```python
from build123d import *

# Parameters (mm, degrees)
F0_R      = 1.778
F1_DEPTH  = 4
F2_R      = 38
F2_R_2    = 34.25
F3_DEPTH  = 15.24
F4_R      = 33.9471
F4_R_2    = 31
F5_DEPTH  = 1.27
F7_DEPTH  = 5.08
F8_R      = 3.81221
F8_R_2    = 3.881316
F8_R_3    = 3.942619
F8_R_4    = 3.925346
F9_DEPTH  = 1.5
F10_R     = 1.778
F11_DEPTH = 25.4


with BuildPart() as f1:
    # F0 (on Top) → F1 (new body)
    with BuildSketch(Plane.XY):
        Polygon((38.268343, -38.268343), (54.11961, 0), (38.268343, 38.268343), (0, 54.11961), (-38.268343, 38.268343), (-54.11961, 0), (-38.268343, -38.268343), (0, -54.11961), align=None)
        with Locations((0, -45.129232)):
            Circle(F0_R, mode=Mode.SUBTRACT)
        with Locations((-45.129232, 0)):
            Circle(F0_R, mode=Mode.SUBTRACT)
        with Locations((45.129232, 0)):
            Circle(F0_R, mode=Mode.SUBTRACT)
        with Locations((0, 45.129232)):
            Circle(F0_R, mode=Mode.SUBTRACT)
    extrude(amount=F1_DEPTH)

    # F2 (on Top) → F3 (join)
    with BuildSketch(Plane.XY):
        Circle(F2_R)
        Circle(F2_R_2, mode=Mode.SUBTRACT)
    extrude(amount=F3_DEPTH)

    # F4 (on face) → F5 (join)
    with BuildSketch(Plane.XY.offset(4)):
        Circle(F4_R)
        Circle(F4_R_2, mode=Mode.SUBTRACT)
    extrude(amount=F5_DEPTH)

    # F6 (on face) → F7 (join)
    with BuildSketch(Plane.XY.offset(4)):
        Polygon((7.838351, 13.74736), (-7.838351, 13.74736), (-7.838351, 11.297162), (-7.838351, 7.838351), (-11.297162, 7.838351), (-13.74736, 7.838351), (-13.74736, -7.838351), (-11.117557, -7.838351), (-7.838351, -7.838351), (-7.838351, -11.117557), (-7.838351, -13.74736), (7.838351, -13.74736), (7.838351, -11.297162), (7.838351, -7.838351), (11.297162, -7.838351), (13.74736, -7.838351), (13.74736, 7.838351), (11.117557, 7.838351), (7.838351, 7.838351), (7.838351, 11.117557), align=None)
        with BuildLine():
            ThreePointArc((-5.298351, 6.12736), (-3.810454, 9.719462), (-0.218351, 11.20736))
            Line((-0.218351, 11.20736), (0.218351, 11.20736))
            ThreePointArc((0.218351, 11.20736), (3.810454, 9.719462), (5.298351, 6.12736))
            Line((5.298351, 6.12736), (5.298351, 5.298351))
            Line((5.298351, 5.298351), (6.12736, 5.298351))
            ThreePointArc((6.12736, 5.298351), (9.719462, 3.810454), (11.20736, 0.218351))
            Line((11.20736, 0.218351), (11.20736, -0.218351))
            ThreePointArc((11.20736, -0.218351), (9.719462, -3.810454), (6.12736, -5.298351))
            Line((6.12736, -5.298351), (5.298351, -5.298351))
            Line((5.298351, -5.298351), (5.298351, -6.12736))
            ThreePointArc((5.298351, -6.12736), (3.810454, -9.719462), (0.218351, -11.20736))
            Line((0.218351, -11.20736), (-0.218351, -11.20736))
            ThreePointArc((-0.218351, -11.20736), (-3.810454, -9.719462), (-5.298351, -6.12736))
            Line((-5.298351, -6.12736), (-5.298351, -5.298351))
            Line((-5.298351, -5.298351), (-6.12736, -5.298351))
            ThreePointArc((-6.12736, -5.298351), (-9.719462, -3.810454), (-11.20736, -0.218351))
            Line((-11.20736, -0.218351), (-11.20736, 0.218351))
            ThreePointArc((-11.20736, 0.218351), (-9.719462, 3.810454), (-6.12736, 5.298351))
            Line((-6.12736, 5.298351), (-5.298351, 5.298351))
            Line((-5.298351, 5.298351), (-5.298351, 6.12736))
        make_face(mode=Mode.SUBTRACT)
    extrude(amount=F7_DEPTH)

    # F8 (on face) → F9 (join)
    with BuildSketch(Plane.XY.offset(4)):
        with Locations((0, 45.151103)):
            Circle(F8_R)
        with Locations((-45.181099, 0)):
            Circle(F8_R_2)
        with Locations((0, -45.120213)):
            Circle(F8_R_3)
        with Locations((45.201581, 0)):
            Circle(F8_R_4)
    extrude(amount=F9_DEPTH)

    # F10 (on face) → F11 (cut)
    with BuildSketch(Plane(origin=(0, 0, 0), x_dir=(1, 0, 0), z_dir=(0, 0, -1))):
        with Locations((45.129232, 0)):
            Circle(F10_R)
        with Locations((0, -45.129232)):
            Circle(F10_R)
        with Locations((-45.129232, 0)):
            Circle(F10_R)
        with Locations((0, 45.129232)):
            Circle(F10_R)
    extrude(amount=-F11_DEPTH, mode=Mode.SUBTRACT)


solid = f1.part
```
The model under review builds one solid part; all positions refer to its coordinate system, in mm. A direction names the side the tool comes from. Coordinates: 2 decimals unless noted, no trailing zeros. Write each loop counter-clockwise with the first axis right and the second up, starting at its lowest first coordinate (ties: lowest second). Pieces come first, ordered by that corner, then holes.
1) We need section B-B on x = 18. State the section outline as (y, z) points, then the cut area to 3 significant figures.
2) We need section A-A on z = 2.75. State the section outline as (x, y) points.
3) We need section C-C on z = 11. State the section outline as (x, y) points, then the cut area to 3 significant figures.
4) Clearance check with flat-ended pins moving along their axes: pin 1 Ø2.5 at (y, z) = (12, 5.5) entering from +X; pin 2 Ø1 at (y, z) = (22.5, 8) entering from +X; pin 3 Ø8 at (x, z) = (6.5, 9.5) entering from -Y; pin 4 Ø6 at (x, y) = (41, -14) entering from -Z. State where each tip first meets the part, or that it passes through.
5) To check wall thickness, follow probe 1 along Y at (x, z) = (0, 3.4); probe 2 along Z at (x, y) = (41.5, -9.5); probe 3 along Y at (x, z) = (8, 8.5). State the ranges of each line that lie inside material, in increasing order.
6) We need section D-D on x = -21. State the section outline as (y, z) points, then the cut area to 3 significant figures.
7) Machinability: for faces 1 (the face through (1, -47, 5.5)), 2 (the face through (46.305, 18.866, 1.972)), 3 (the face through (48.83, -1.5, 4.74)), which of the approach directions +Z, -Z, +X, -X, +Y, -Y give a long, thin tool a straight path to every point of the face, cutting with its end or side? Answer none if there is none.
Answer list:
1. outline: (-46.66, 0) - (46.66, 0) - (46.66, 4) - (33.47, 4) - (33.47, 15.24) - (29.14, 15.24) - (29.14, 4) - (28.78, 4) - (28.78, 5.27) - (25.24, 5.27) - (25.24, 4) - (-25.24, 4) - (-25.24, 5.27) - (-28.78, 5.27) - (-28.78, 4) - (-29.14, 4) - (-29.14, 15.24) - (-33.47, 15.24) - (-33.47, 4) - (-46.66, 4) - close
1. area: 480 mm2
2. outline: (-54.12, 0) - (-38.27, -38.27) - (0, -54.12) - (38.27, -38.27) - (54.12, 0) - (38.27, 38.27) - (0, 54.12) - (-38.27, 38.27) - close; hole circle Ø3.56 at (-45.13, 0); hole circle Ø3.56 at (0, -45.13); hole circle Ø3.56 at (0, 45.13); hole circle Ø3.56 at (45.13, 0)
3. outline: circle Ø76 at (0, 0); hole circle Ø68.5 at (0, 0)
3. area: 851 mm2
4. pin 1: stops at x = 36.45
4. pin 2: stops at x = 30.98
4. pin 3: stops at y = -37.92
4. pin 4: stops at z = 0
5. probe 1: y = -54.12 to -46.91, -43.35 to 43.35, 46.91 to 54.12
5. probe 2: z = 0 to 4
5. probe 3: y = -37.15 to -33.3, -7.84 to -4.94, 4.94 to 7.84, 33.3 to 37.15
6. outline: (-45.42, 0) - (45.42, 0) - (45.42, 4) - (31.67, 4) - (31.67, 15.24) - (27.06, 15.24) - (27.06, 4) - (26.67, 4) - (26.67, 5.27) - (22.8, 5.27) - (22.8, 4) - (-22.8, 4) - (-22.8, 5.27) - (-26.67, 5.27) - (-26.67, 4) - (-27.06, 4) - (-27.06, 15.24) - (-31.67, 15.24) - (-31.67, 4) - (-45.42, 4) - close
6. area: 477 mm2
7. face 1: +Z, +X, -X, -Y
7. face 2: +Z, -Z, +X, +Y
7. face 3: +Z
